Source: CAD feature listing. Evaluate the final solid. Frame: model axes, mm. Face numbers are marked on the shaded views. A direction names the side the tool comes from. Give positions to 0.01 mm unless a question says otherwise; leave off trailing zeros. Order: outer loops, then holes, each group sorted by start corner. A loop starts at its lowest first (then second) coordinate and runs counter-clockwise, first axis right, second up. Notation, with made-up numbers: M 53.25,73.25 L 106.25,73.25 A18 cw 106.25,107.25 Z; hole C 70.25,65 d11. An arc over 180 degrees is marked long. Answer in a Markdown table with one row per item. Add a question column.
(1) Pin query (flat end, axial travel): P1, Ø10, axis at x = 2.5, z = -52, coming from the +Y side; P2, Ø4, axis at x = 6.5, z = 36.5, coming from the +Y side; P3, Ø5, axis at x = -6, y = 7.5, coming from the +Z side. Return the tip coordinate at first contact, or that it passes through.
(2) Set-up query: the marked faces 1, 2 and 3. Return all of +Z, -Z, +X, -X, +Y, -Y with unobstructed straight access to the full face (end or side cutting, diameter ignored); none if empty.
(3) Section query C-C, the plane z = 24. Return loops of the section in (x, y).
(4) Material intervals for line 1 along Y through (x, z) = (0, 8.5); line 2 along Y through (x, z) = (0, 37), sorted ascending.
(5) Section query A-A, the plane x = 0. Return loops of the section in (y, z), plus the area to 3 significant figures.
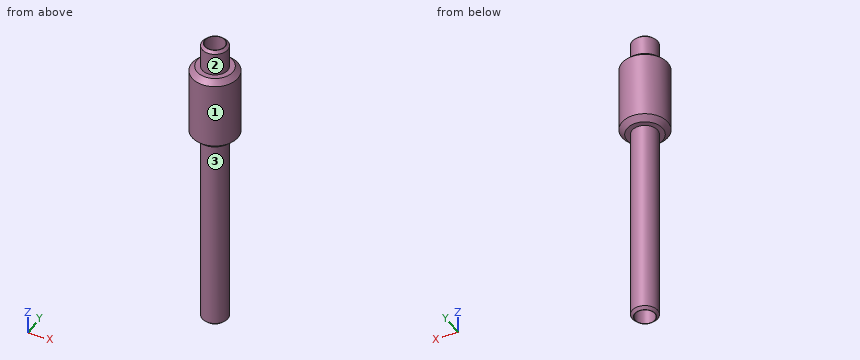
from build123d import *

# Parameters (mm, degrees)
F2_SIZE  = 2.54
F3_R     = 4.880462
F6_DEPTH = 152.401
F4_SIZE  = 1.27
F7_SIZE  = 2.54
F5_SIZE  = 1.27


with BuildPart() as f1:
    # F0 (on Front) → F1 (revolve)
    with BuildSketch(Plane.XZ):
        Polygon((0, -76.2), (6.35, -76.2), (6.35, 25.4), (11.43, 25.4), (11.43, 63.5), (6.35, 63.5), (6.35, 76.2), (0, 76.2), align=None)
    revolve(axis=Axis((0, 0, -2.097856), (0, 0, -1)))

    # F2
    f2_edges = [f1.edges().sort_by_distance(p)[0] for p in [
        (-11.43, 0, 25.4),
    ]]
    chamfer(f2_edges, length=F2_SIZE)

    # F3 (on face) → F6 (cut, through all)
    with BuildSketch(Plane(origin=(0, 0, -76.2), x_dir=(1, 0, 0), z_dir=(0, 0, -1))):
        Circle(F3_R)
    extrude(amount=-F6_DEPTH, mode=Mode.SUBTRACT)

    # F4
    f4_edges = [f1.edges().sort_by_distance(p)[0] for p in [
        (-6.35, 0, 76.2),
    ]]
    chamfer(f4_edges, length=F4_SIZE)

    # F7
    f7_edges = [f1.edges().sort_by_distance(p)[0] for p in [
        (-11.43, 0, 63.5),
    ]]
    chamfer(f7_edges, length=F7_SIZE)

    # F5
    f5_edges = [f1.edges().sort_by_distance(p)[0] for p in [
        (-6.35, 0, -76.2),
    ]]
    chamfer(f5_edges, length=F5_SIZE)


solid = f1.part
Values follow:
| question | item | result |
|---|---|---|
| 1 | P1 | stops at y = 6.35 |
| 1 | P2 | stops at y = 10.51 |
| 1 | P3 | stops at z = 63.5 |
| 2 | face 1 | +Z, -Z |
| 2 | face 2 | +Z |
| 2 | face 3 | -Z |
| 3 | outline | C 0,0 d12.7; hole C 0,0 d9.76 |
| 4 | line 1 | y = -6.35 to -4.88, 4.88 to 6.35 |
| 4 | line 2 | y = -11.43 to -4.88, 4.88 to 11.43 |
| 5 | outline | M -11.43,27.94 L -8.89,25.4 L -6.35,25.4 L -6.35,-74.93 L -5.08,-76.2 L -4.88,-76.2 L -4.88,76.2 L -5.08,76.2 L -6.35,74.93 L -6.35,63.5 L -8.89,63.5 L -11.43,60.96 Z; M 4.88,-76.2 L 5.08,-76.2 L 6.35,-74.93 L 6.35,25.4 L 8.89,25.4 L 11.43,27.94 L 11.43,60.96 L 8.89,63.5 L 6.35,63.5 L 6.35,74.93 L 5.08,76.2 L 4.88,76.2 Z |
| 5 | area | 819 mm² |
